Source: three-view drawing plus pictorial views. Frame: mm from the lowest corner of the part. A direction names the side the tool comes from. Give positions to 0.01 mm unless a question says otherwise; leave off trailing zeros. Write each loop counter-clockwise with the first axis right and the second up, starting at its lowest first coordinate (ties: lowest second). Pieces come first, ordered by that corner, then holes.
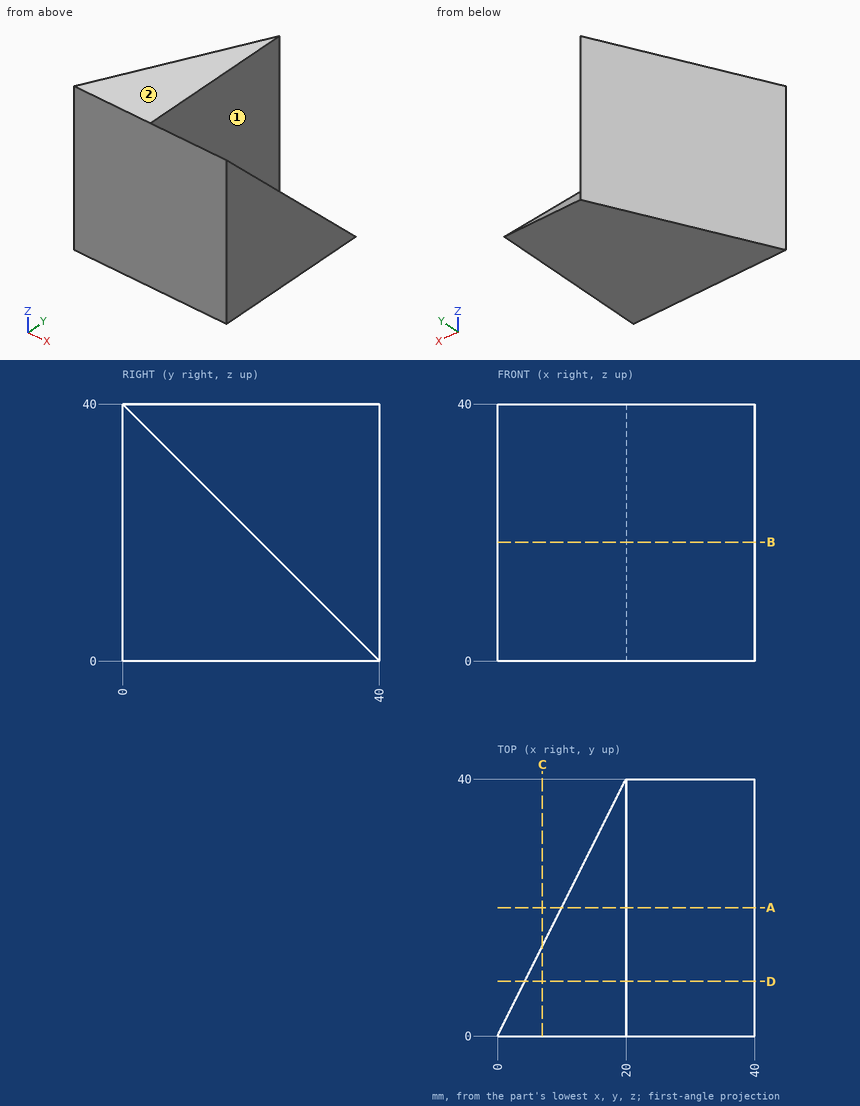
Q1. Pin query (flat end, axial travel): P1, Ø8, axis at x = 31, y = 10.5, coming from the +Z side; P2, Ø5, axis at x = 4.5, z = 10.5, coming from the +Y side; P3, Ø8, axis at x = 15, z = 14.5, coming from the +Y side; P4, Ø12, axis at y = 27.5, z = 15, coming from the +X side. Return the tip coordinate at first contact, or that it passes through.
Filled sheet:
P1: stops at z = 33.5
P2: stops at y = 14
P3: stops at y = 38
P4: stops at x = 40
Q2. Ray query, line 1 along Z through (x, y) = (33, 24.5); line 2 along Z through (x, y) = (22.5, 3); line 3 along Y through (x, z) = (5, 34.5). Return the intervals inside material, ascending.
Filled sheet:
line 1: z = 0 to 15.5
line 2: z = 0 to 37
line 3: y = 0 to 10
Q3. Access query for the marked faces 1 and 2. Directions: +Z, -Z, +X, -X, +Y, -Y. A direction counts if a zero-diameter tool reaches every point of the face in a straight line with its end or side. Return the directions, or none.
Filled sheet:
face 1: +Z, +X, +Y
face 2: +Z, +X, -X, +Y, -Y
Q4. Section A-A on y = 20. Output: boundary loops of the cut face in (x, z), plus the area to 3 significant figures.
Filled sheet:
outline: (10, 0) - (40, 0) - (40, 20) - (20, 20) - (20, 40) - (10, 40) - close
area: 800 mm2
Q5. Section B-B on z = 18.5. Output: boundary loops of the cut face in (x, y), plus the area to 3 significant figures.
Filled sheet:
outline: (0, 0) - (40, 0) - (40, 21.5) - (20, 21.5) - (20, 40) - close
area: 830 mm2
Q6. Section D-D on y = 8.5. Output: boundary loops of the cut face in (x, z), plus the area to 3 significant figures.
Filled sheet:
outline: (4.25, 0) - (40, 0) - (40, 31.5) - (20, 31.5) - (20, 40) - (4.25, 40) - close
area: 1,260 mm2
Q7. Section C-C on x = 7. Output: boundary loops of the cut face in (y, z), plus the area to 3 significant figures.
Filled sheet:
outline: (0, 0) - (14, 0) - (14, 40) - (0, 40) - close
area: 560 mm2
